Part print with two shaded views. Sizes in mm from the minimum x, y, z corner. A direction names the side the tool comes from. Round coordinates to 2 decimals unless told otherwise and drop trailing zeros. Write each loop counter-clockwise with the first axis right and the second up, starting at its lowest first coordinate (ties: lowest second). Pieces come first, ordered by that corner, then holes. Notation, with made-up numbers: (29.5, 50.5) -> (40.5, 50.5) arc R32 cw to (40.5, 79.5) -> close; hole circle Ø7 at (5.25, 48). An arc over 180 degrees is marked (long way). Put each result on its own line as item: value. Start each with the question number.
1. Drill centre lines: line 1 (Y direction, x = 12, z = 83.75); line 2 (Y direction, x = 35, z = 81); line 3 (X direction, y = 113.5, z = 48). Where is each one in solid material? Low to high. Write a range as from..to.
2. 3-axis set-ups, long thin cutter, end or side, ignore diameter. For the marked faces 4, 5 and 6: which of +Z, -Z, +X, -X, +Y, -Y reach the whole face in a straight line?
3. Saw through at D-D on y = 14. List the corners of the cut face in (x, z).
4. Saw through at B-B on x = 35.5. List the corners of the cut face in (y, z).
5. Flat gauge pins, fed straight in: P1, Ø3, axis at x = 12, y = 134, coming from the -Z side; P2, Ø12, axis at x = 15.5, z = 71, coming from the -Y side; P3, Ø6, axis at x = 59, y = 134, coming from the +Z side; P4, Ø17, axis at x = 43, y = 120.5, coming from the -Z side. Where does each tip first touch, or does it go through?
6. Saw through at C-C on z = 80.5. List the corners of the cut face in (x, y).
7. Pull direction X, two halves, no side cores. Call the marked faces 1, 2 and 3: pulls with the +X half, pulls with the -X half, needs draft (parallel to the pull), parting line crosses it, or undercut.
8. Saw through at A-A on y = 87. List the corners of the cut face in (x, z), and give its area (3 significant figures).
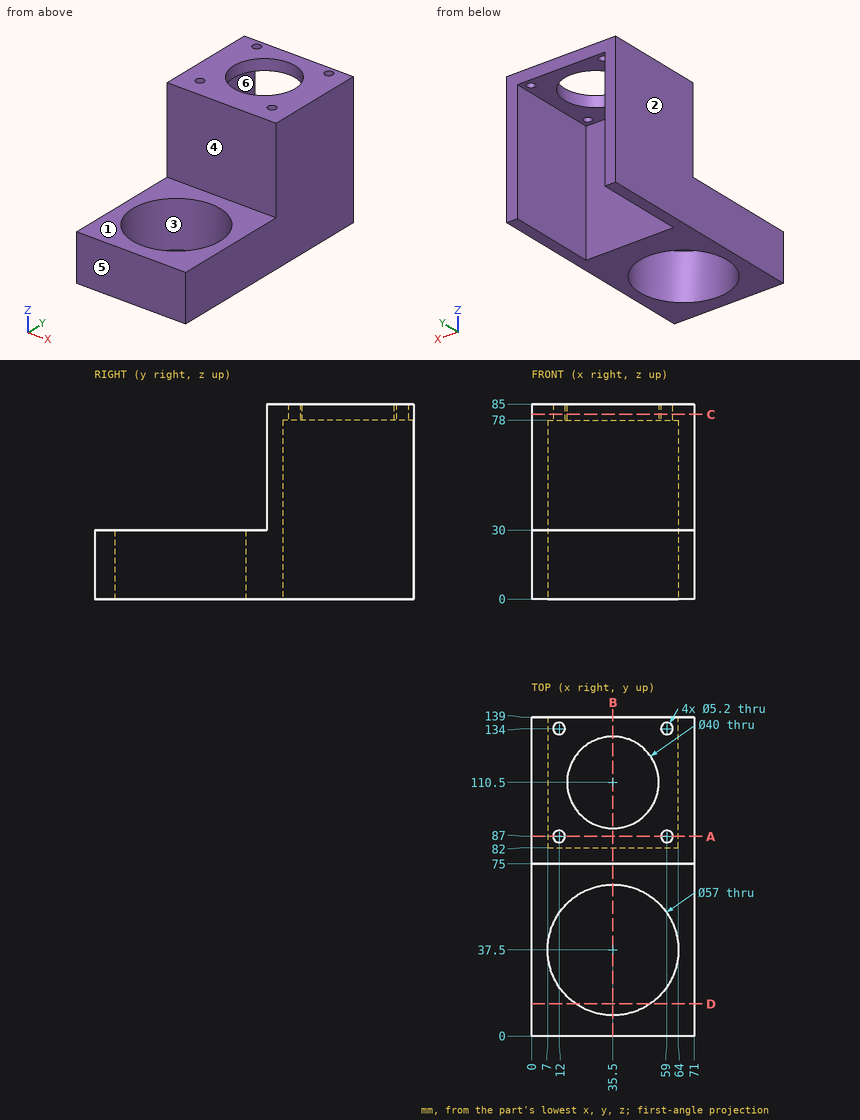
Return value:
1. line 1: y = 75..84.4, 89.6..131.4, 136.6..139
1. line 2: y = 75..90.51, 130.49..139
1. line 3: x = 0..7, 64..71
2. face 4: +Z, +X, -X, -Y
2. face 5: +Z, -Z, +X, -X, -Y
2. face 6: -Z, +Y
3. outline: (0, 0) -> (19.38, 0) -> (19.38, 30) -> (0, 30) -> close; (51.62, 0) -> (71, 0) -> (71, 30) -> (51.62, 30) -> close
4. outline: (0, 0) -> (9, 0) -> (9, 30) -> (0, 30) -> close; (66, 0) -> (82, 0) -> (82, 78) -> (90.5, 78) -> (90.5, 85) -> (75, 85) -> (75, 30) -> (66, 30) -> close; (130.5, 78) -> (139, 78) -> (139, 85) -> (130.5, 85) -> close
5. P1: passes through
5. P2: stops at y = 75
5. P3: stops at z = 85
5. P4: stops at z = 78
6. outline: (0, 75) -> (71, 75) -> (71, 139) -> (0, 139) -> close; hole circle Ø5.2 at (12, 87); hole circle Ø5.2 at (12, 134); hole circle Ø40 at (35.5, 110.5); hole circle Ø5.2 at (59, 87); hole circle Ø5.2 at (59, 134)
7. face 1: needs draft
7. face 2: pulls with the -X half
7. face 3: undercut
8. outline: (0, 0) -> (7, 0) -> (7, 78) -> (9.4, 78) -> (9.4, 85) -> (0, 85) -> close; (14.6, 78) -> (56.4, 78) -> (56.4, 85) -> (14.6, 85) -> close; (61.6, 78) -> (64, 78) -> (64, 0) -> (71, 0) -> (71, 85) -> (61.6, 85) -> close
8. area: 1,520 mm^2
